The model under review builds one solid part; all positions refer to its coordinate system, in mm. Round coordinates to 2 decimals unless told otherwise and drop trailing zeros. Order: outer loops, then holes, each group sorted by start corner. A loop starts at its lowest first (then second) coordinate and runs counter-clockwise, first axis right, second up.
1) To check wall thickness, follow L1, parallel to Y at x = 0, z = 2; L2, parallel to X at y = -6, z = 2; L3, parallel to Y at x = -2, z = 4.75. State the ranges of each line that lie inside material, in increasing order.
2) Clearance check with flat-ended pins moving along their axes: P1, Ø1.5, axis at x = 2, z = 5.5, coming from the +Y side; P2, Ø3, axis at x = -8, z = 3, coming from the +Y side. State where each tip first meets the part, or that it passes through.
3) Consider section A-A (z = 2.25). Give the boundary of the cut face in (x, y).
from build123d import *

# Parameters (mm, degrees)
RESSALTO_EXTRUS_O1_DEPTH                 = 6.4
ESBO_O2_OUTSIDE_W                        = 151.914
ESBO_O2_OUTSIDE_H                        = 156.4
ESBO_O2_OUTSIDE_R                        = 14.5
CORTE_EXTRUS_O1_DEPTH                    = 15
CORTE_EXTRUS_O1_DRAFT                    = -75
ESBO_O3_OUTSIDE_W                        = 151.914
ESBO_O3_OUTSIDE_H                        = 156.4
ESBO_O3_OUTSIDE_R                        = 14.5
CORTE_EXTRUS_O2_DEPTH                    = 15
CORTE_EXTRUS_O2_DRAFT                    = -75
BROCA_DE_ROSQUEAR_PARA_TARRAXA_DE_M221_D = 19.5


with BuildPart() as part:
    # Esboço1 → Ressalto-extrusão1 (new body)
    with BuildSketch(Plane.XY):
        Polygon((0, 16.743157806), (-14.5, 8.371578903), (-14.5, -8.371578903), (0, -16.743157806), (14.5, -8.371578903), (14.5, 8.371578903), align=None)
    extrude(amount=RESSALTO_EXTRUS_O1_DEPTH)


with BuildPart() as corte_extrus_o1_tool:
    # Esboço2 outside → Corte-extrusão1 (with draft: the straight prism first)
    with BuildSketch(Plane.XY.offset(6.4)):
        Rectangle(ESBO_O2_OUTSIDE_W, ESBO_O2_OUTSIDE_H)
        Circle(ESBO_O2_OUTSIDE_R, mode=Mode.SUBTRACT)
    extrude(amount=-CORTE_EXTRUS_O1_DEPTH)
    # Corte-extrusão1: the draft: its side faces are tilted about the plane it starts from
    corte_extrus_o1_sides = [corte_extrus_o1_tool.faces().sort_by_distance(p)[0] for p in [
        (0, -78.2, -1.1),
        (75.957, 0, -1.1),
        (0, 78.2, -1.1),
        (-75.957, 0, -1.1),
        (-14.5, 0, -1.1),
    ]]
    draft(corte_extrus_o1_sides, Plane.XY.offset(6.4), CORTE_EXTRUS_O1_DRAFT)


with BuildPart() as part_1:
    add(part.part)

    # Corte-extrusão1: cut by corte_extrus_o1_tool
    add(corte_extrus_o1_tool.part, mode=Mode.SUBTRACT)


with BuildPart() as corte_extrus_o2_tool:
    # Esboço3 outside → Corte-extrusão2 (with draft: the straight prism first)
    with BuildSketch(Plane(origin=(0, 0, 0), x_dir=(-1, 0, 0), z_dir=(0, 0, -1))):
        Rectangle(ESBO_O3_OUTSIDE_W, ESBO_O3_OUTSIDE_H)
        Circle(ESBO_O3_OUTSIDE_R, mode=Mode.SUBTRACT)
    extrude(amount=-CORTE_EXTRUS_O2_DEPTH)
    # Corte-extrusão2: the draft: its side faces are tilted about the plane it starts from
    corte_extrus_o2_sides = [corte_extrus_o2_tool.faces().sort_by_distance(p)[0] for p in [
        (0, -78.2, 7.5),
        (-75.957, 0, 7.5),
        (0, 78.2, 7.5),
        (75.957, 0, 7.5),
        (14.5, 0, 7.5),
    ]]
    draft(corte_extrus_o2_sides, Plane(origin=(0, 0, 0), x_dir=(-1, 0, 0), z_dir=(0, 0, -1)), CORTE_EXTRUS_O2_DRAFT)


with BuildPart() as part_2:
    add(part_1.part)

    # Corte-extrusão2: cut by corte_extrus_o2_tool
    add(corte_extrus_o2_tool.part, mode=Mode.SUBTRACT)

    # Broca de rosquear para tarraxa de M221 (through all)
    with Locations(Plane(origin=(0, 0, 0), x_dir=(-1, 0, 0), z_dir=(0, 0, -1))):
        with Locations((0, 0)):
            Hole(BROCA_DE_ROSQUEAR_PARA_TARRAXA_DE_M221_D / 2)


solid = part_2.part
Answer below:
1. L1: y = -16.74 to -9.75, 9.75 to 16.74
1. L2: x = -14.5 to -7.69, 7.69 to 14.5
1. L3: y = -15.59 to -9.54, 9.54 to 15.59
2. P1: stops at y = 16.02
2. P2: stops at y = 12.99
3. outline: (-14.5, -8.37) - (0, -16.74) - (14.5, -8.37) - (14.5, 8.37) - (0, 16.74) - (-14.5, 8.37) - close; hole circle Ø19.5 at (0, 0)
